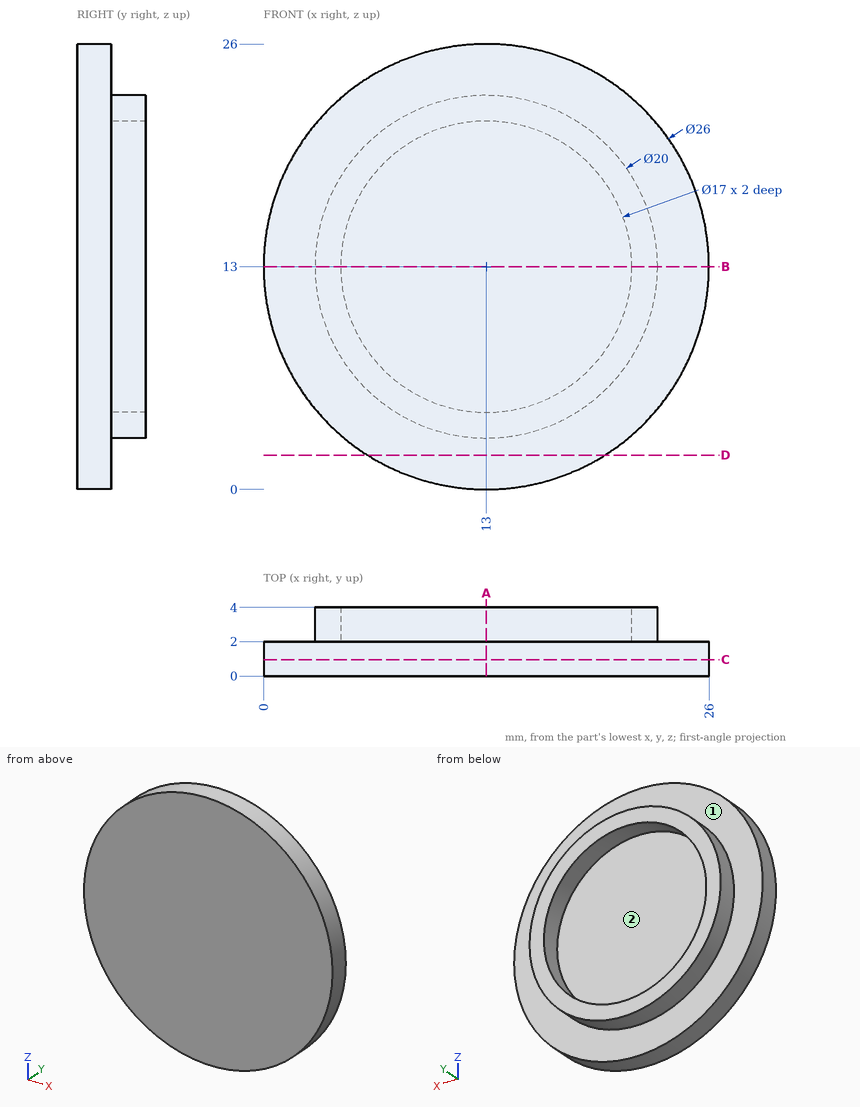
Job drawing, mm, ordinate dimensions from the low corner. One solid piece. Coordinates: 2 decimals unless noted, no trailing zeros. Order: outer loops, then holes, each group sorted by start corner. A loop starts at its lowest first (then second) coordinate and runs counter-clockwise, first axis right, second up. Notation, with made-up numbers: (33.25, 45) - (45.25, 45) arc R15 cw to (45.25, 74) - close; hole circle Ø3 at (31, 7). An arc over 180 degrees is marked (long way). Return JSON: item names as keys, results as strings. Group by question number.
1) Saw through at A-A, the plane x = 13. Write the cut outline in (y, z).
2) Saw through at D-D, the plane z = 2. Write the cut outline in (x, y), plus the area to 3 significant figures.
3) Mould opens along X. For the marked faces 1 and 2 say: released by +X, released by -X, zero draft, split by the parting line, or undercut.
4) Saw through at C-C, the plane y = 0.95. Write the cut outline in (x, z), plus the area to 3 significant figures.
5) Probe line 1 (Z direction, x = 13, y = 2.7); line 2 (Y direction, x = 18, z = 3.25); line 3 (X direction, y = 3.6, z = 17.5). List the from-to ranges inside material, lowest first. Write a range as from..to.
6) Saw through at B-B, the plane z = 13. Write the cut outline in (x, y).
7) Flat gauge pin, fed straight in: P1, Ø13.5, axis at x = 13, z = 13, coming from the +Y side. Where does the tip first touch, or does it go through?
Values found:
{
 "1": {"outline": "(0, 0) - (2, 0) - (2, 3) - (4, 3) - (4, 4.5) - (2, 4.5) - (2, 21.5) - (4, 21.5) - (4, 23) - (2, 23) - (2, 26) - (0, 26) - close"},
 "2": {"outline": "(6.07, 0) - (19.93, 0) - (19.93, 2) - (6.07, 2) - close", "area": "27.7 mm²"},
 "3": {"face 1": "zero draft", "face 2": "undercut"},
 "4": {"outline": "circle Ø26 at (13, 13)", "area": "531 mm²"},
 "5": {"line 1": "z = 3..4.5, 21.5..23", "line 2": "y = 0..2", "line 3": "x = 4.07..5.79, 20.21..21.93"},
 "6": {"outline": "(0, 0) - (26, 0) - (26, 2) - (23, 2) - (23, 4) - (21.5, 4) - (21.5, 2) - (4.5, 2) - (4.5, 4) - (3, 4) - (3, 2) - (0, 2) - close"},
 "7": {"P1": "stops at y = 2"}
}
